Autodesk Inventor part; units mm, degrees
ref_plane "YZ Plane" through (0, 0, 0) normal (1, 0, 0) x (0, 1, 0)
ref_plane "XZ Plane" through (0, 0, 0) normal (0, 1, 0) x (-1, 0, 0)
ref_plane "XY Plane" through (0, 0, 0) normal (0, 0, 1) x (1, 0, 0)
sketch "Sketch1" plane through (0, 0, 0) normal (0, 1, 0) x (-1, 0, 0)
  line L0 (457.2, 330.2) -> (-457.2, 330.2)
  line L1 (-457.2, 330.2) -> (-457.2, -330.2)
  line L2 (-457.2, -330.2) -> (457.2, -330.2)
  line L3 (457.2, -330.2) -> (457.2, 330.2)
  line L4 (457.2, 330.2) -> (-457.2, -330.2) construction
  line L5 (-457.2, 330.2) -> (457.2, -330.2) construction
  line L6 (-431.8, -304.8) -> (-431.8, 304.8)
  line L7 (-431.8, 304.8) -> (431.8, 304.8)
  line L8 (431.8, 304.8) -> (431.8, -304.8)
  line L9 (431.8, -304.8) -> (-431.8, -304.8)
  line L10 (-431.8, 152.4) -> (431.8, 152.4)
  line L11 (431.8, 152.4) -> (431.8, 127)
  line L12 (431.8, 127) -> (-431.8, 127)
  line L13 (-431.8, 127) -> (-431.8, 152.4)
  line L14 (431.8, -127) -> (-431.8, -127)
  line L15 (-431.8, -127) -> (-431.8, -152.4)
  line L16 (-431.8, -152.4) -> (431.8, -152.4)
  line L17 (431.8, -152.4) -> (431.8, -127)
  point P0 (0, 0)
  point P1 (0, -152.4)
  dimension "d0" = 914.4
  dimension "d1" = 660.4
  dimension "d2" = 25.4
  dimension "d3" = 25.4
  dimension "d4" = 25.4
  dimension "d5" = 152.4
  dimension "d6" = 152.4
extrude "Extrusion1" add sketch "Sketch1" along normal blind 25.4 contours L3 L2 L1 L0 | L6 L14 L8 L16 | L6 L10 L8 L12
sketch "Sketch2" plane through (0, 25.4, 0) normal (0, 1, 0) x (1, 0, 0)
  line L0 (-457.2, 330.2) -> (-457.2, -330.2)
  line L1 (431.8, -304.8) -> (-431.8, -304.8)
  line L2 (-457.2, -330.2) -> (-431.8, -330.2)
  line L3 (-431.8, -330.2) -> (-431.8, -304.8)
  line L4 (-431.8, -304.8) -> (-457.2, -304.8)
  line L5 (-457.2, -304.8) -> (-457.2, -330.2)
  line L6 (457.2, 330.2) -> (-457.2, 330.2)
  line L7 (-431.8, 304.8) -> (431.8, 304.8)
  line L8 (-457.2, 330.2) -> (-431.8, 330.2)
  line L9 (-431.8, 330.2) -> (-431.8, 304.8)
  line L10 (-431.8, 304.8) -> (-457.2, 304.8)
  line L11 (-457.2, 304.8) -> (-457.2, 330.2)
  line L12 (457.2, -330.2) -> (457.2, 330.2)
  line L13 (457.2, 330.2) -> (431.3742, 330.2)
  line L14 (431.3742, 330.2) -> (431.3742, 304.8)
  line L15 (431.3742, 304.8) -> (457.2, 304.8)
  line L16 (457.2, 304.8) -> (457.2, 330.2)
  line L17 (457.2, -330.2) -> (431.8, -330.2)
  line L18 (431.8, -330.2) -> (431.8, -304.8)
  line L19 (431.8, -304.8) -> (457.2, -304.8)
  line L20 (457.2, -304.8) -> (457.2, -330.2)
  point P0 (0, 0)
extrude "Extrusion2" add sketch "Sketch2" along normal blind 457.2 contours L6 L9 L10 L0 | L4 L3 L2 L0 | L6 L12 L15 L7 L14 | L19 L12 L17 L18
sketch "Sketch3" plane through (0, 482.6, 0) normal (0, 1, 0) x (1, 0, 0)
  line L0 (431.8, -127) -> (-431.8, -127)
  line L1 (-431.8, -127) -> (-431.8, 127)
  line L2 (-431.8, 127) -> (431.8, 127)
  line L3 (431.8, 127) -> (431.8, -127)
  line L4 (457.2, 304.8) -> (431.8, 304.8)
  line L5 (431.8, 304.8) -> (431.8, 152.4)
  line L6 (431.8, 152.4) -> (-431.8, 152.4)
  line L7 (-431.8, 152.4) -> (-431.8, 304.8)
  line L8 (-431.8, 304.8) -> (-457.2, 304.8)
  line L9 (-457.2, 304.8) -> (-457.2, -304.8)
  line L10 (-457.2, -304.8) -> (-431.8, -304.8)
  line L11 (-431.8, -304.8) -> (-431.8, -152.4)
  line L12 (-431.8, -152.4) -> (431.8, -152.4)
  line L13 (431.8, -152.4) -> (431.8, -304.8)
  line L14 (431.8, -304.8) -> (457.2, -304.8)
  line L15 (457.2, -304.8) -> (457.2, 304.8)
  line L16 (431.3742, 304.8) -> (431.3742, 330.2)
  line L17 (431.3742, 330.2) -> (-431.8, 330.2)
  line L18 (-431.8, 330.2) -> (-431.8, 304.8)
  line L19 (-431.8, 304.8) -> (431.3742, 304.8)
  line L20 (431.8, -330.2) -> (431.8, -304.8)
  line L21 (431.8, -304.8) -> (-431.8, -304.8)
  line L22 (-431.8, -304.8) -> (-431.8, -330.2)
  line L23 (-431.8, -330.2) -> (431.8, -330.2)
  line L24 (-431.8, -330.2) -> (-431.8, -304.8)
  line L25 (-431.8, -304.8) -> (-457.2, -304.8)
  line L26 (-457.2, -304.8) -> (-457.2, -330.2)
  line L27 (-457.2, -330.2) -> (-431.8, -330.2)
  line L28 (-431.8, 304.8) -> (-431.8, 330.2)
  line L29 (-431.8, 330.2) -> (-457.2, 330.2)
  line L30 (-457.2, 330.2) -> (-457.2, 304.8)
  line L31 (-457.2, 304.8) -> (-431.8, 304.8)
  line L32 (457.2, 304.8) -> (457.2, 330.2)
  line L33 (457.2, 330.2) -> (431.3742, 330.2)
  line L34 (431.3742, 330.2) -> (431.3742, 304.8)
  line L35 (431.3742, 304.8) -> (457.2, 304.8)
  line L36 (457.2, -304.8) -> (431.8, -304.8)
  line L37 (431.8, -330.2) -> (457.2, -330.2)
  line L38 (457.2, -330.2) -> (457.2, -304.8)
  line L39 (457.2, -304.8) -> (431.8, -304.8)
  line L40 (431.8, -304.8) -> (431.8, -330.2)
  line L41 (431.8, -152.4) -> (431.8, -304.8)
  line L42 (431.8, -152.4) -> (431.8, 152.4)
  line L43 (431.8, 127) -> (431.8, -127)
  line L44 (-431.8, -152.4) -> (-431.8, 152.4)
  point P0 (0, 0)
  point P1 (431.8, 127)
extrude "Extrusion3" add sketch "Sketch3" along normal blind 25.4 contours L3 L42 L5 L4 L15 L14 L13 | L44 L11 L10 L9 L8 L7 L1 | L14 L38 L37 L20 | L20 L23 L22 L21 | L22 L27 L26 L10 | L35 L16 L33 L32 L4 | L8 L30 L29 L18 | L18 L17 L16 L19
properties part number "Chassis"
Check sheet for the modelled part. Datum: model origin and axes. Units: mm. A direction names the side the tool comes from. Round coordinates to 2 decimals unless told otherwise and drop trailing zeros. Loops run counter-clockwise (first coordinate to the right, second up) from the corner with the lowest first, then second, coordinate; pieces in that order, holes last. Notation, with made-up numbers: (17, 28) -> (30, 28) arc R16 ccw to (30, 41) -> close; hole circle Ø3 at (16.5, -38). An arc over 180 degrees is marked (long way). Write item = value, one per line. Start each with the question number.
1) Gauge pin test, flat end, axial feed: pin 1 Ø20.5 at (x, z) = (-444, 146) entering from -Y. Record the tip position at first contact, or that the pin passes through.
2) Release check for a two-part mould opening along Y. For faces 5 (the flat face through (-6, 482.6, 317)), 6 (the flat face through (431.8, 13, -2)), 7 (the flat face through (36, 0, -145)), 8 (the flat face through (-444, 251, -304.8)) record: released by +Y, released by -Y, zero draft, split by the parting line, or undercut.
3) Sectioned sample at A-A, the plane y = 367. Record the cut outline in (x, z), plus the area to 3 significant figures.
4) Thickness scan on probe 1 along Y at (x, z) = (66, -145). Record the ranges inside material, lowest first.
5) Set-up check for faces 1 (the flat face through (36, 25.4, -134)), 2 (the flat face through (431.8, 13, 228)), 3 (the flat face through (-431.8, 251, 318)), 4 (the flat face through (-431.8, 495, 4)): record each of +Z, -Z, +X, -X, +Y, -Y from which the full face is reachable in a straight line by a thin tool's end or side.
6) Sectioned sample at B-B, the plane z = 243. Record the cut outline in (x, y), plus the area to 3 significant figures.
7) Sectioned sample at C-C, the plane x = 302.5. Record the cut outline in (y, z), plus the area to 3 significant figures.
Results are:
q1.pin_1 = 0
q2.face_5 = undercut
q2.face_6 = zero draft
q2.face_7 = released by -Y
q2.face_8 = undercut
q3.outline = (-457.2, -330.2) -> (-431.8, -330.2) -> (-431.8, -304.8) -> (-457.2, -304.8) -> close; (-457.2, 304.8) -> (-431.8, 304.8) -> (-431.8, 330.2) -> (-457.2, 330.2) -> close; (431.37, -330.2) -> (457.2, -330.2) -> (457.2, -304.8) -> (431.37, -304.8) -> close; (431.8, 304.8) -> (457.2, 304.8) -> (457.2, 330.2) -> (431.8, 330.2) -> close
q3.area = 2,590 mm^2
q4.probe_1 = 0 to 25.4
q5.face_1 = +X, -X
q5.face_2 = +Y, -Y
q5.face_3 = +Z, -Z
q5.face_4 = +Y
q6.outline = (-457.2, 0) -> (-431.8, 0) -> (-431.8, 25.4) -> (-457.2, 25.4) -> close; (-457.2, 482.6) -> (-431.8, 482.6) -> (-431.8, 508) -> (-457.2, 508) -> close; (431.8, 0) -> (457.2, 0) -> (457.2, 25.4) -> (431.8, 25.4) -> close; (431.8, 482.6) -> (457.2, 482.6) -> (457.2, 508) -> (431.8, 508) -> close
q6.area = 2,580 mm^2
q7.outline = (0, -330.2) -> (25.4, -330.2) -> (25.4, -304.8) -> (0, -304.8) -> close; (0, -152.4) -> (25.4, -152.4) -> (25.4, -127) -> (0, -127) -> close; (0, 127) -> (25.4, 127) -> (25.4, 152.4) -> (0, 152.4) -> close; (0, 304.8) -> (25.4, 304.8) -> (25.4, 330.2) -> (0, 330.2) -> close; (482.6, -330.2) -> (508, -330.2) -> (508, -304.8) -> (482.6, -304.8) -> close; (482.6, 304.8) -> (508, 304.8) -> (508, 330.2) -> (482.6, 330.2) -> close
q7.area = 3,870 mm^2
